from build123d import *

# Parameters (mm, degrees)
F1_DEPTH = 0.6
F3_DEPTH = 1.201


# Not quite as in the source:
# - a feature names something its author has since deleted; it is built from what else it names


with BuildPart() as f1:
    # F0 (on Top) → F1 (new body, symmetric)
    with BuildSketch(Plane.XY):
        Polygon((56, 120), (0, 120), (0, 106), (0, 0), (56, 0), (56, 16), (56, 106), align=None)
        with BuildLine():
            ThreePointArc((62, 100), (57.7573593129, 101.7573593129), (56, 106))
            Line((56, 106), (56, 16))
            ThreePointArc((56, 16), (57.7573593129, 20.2426406871), (62, 22))
            Line((62, 22), (67.5, 22))
            Line((67.5, 22), (67.5, 100))
            Line((67.5, 100), (62, 100))
        make_face()
    extrude(amount=F1_DEPTH, both=True)

    # F2 (on face) → F3 (cut, through all)
    with BuildSketch(Plane.XY.offset(0.6)):
        with BuildLine():
            Line((6, 103), (6, 104.5))
            Line((6, 104.5), (7.5, 104.5))
            ThreePointArc((7.5, 104.5), (4.9393398282, 105.5606601718), (6, 103))
        make_face()
        with BuildLine():
            Line((7.5, 104.5), (6, 104.5))
            Line((6, 104.5), (6, 103))
            ThreePointArc((6, 103), (7.0606601718, 103.4393398282), (7.5, 104.5))
        make_face()
        with BuildLine():
            ThreePointArc((51.5, 104.5), (50, 106), (48.5, 104.5))
            Line((48.5, 104.5), (50, 104.5))
            Line((50, 104.5), (50, 103))
            ThreePointArc((50, 103), (51.0606601718, 103.4393398282), (51.5, 104.5))
        make_face()
        with BuildLine():
            Line((50, 104.5), (48.5, 104.5))
            ThreePointArc((48.5, 104.5), (48.9393398282, 103.4393398282), (50, 103))
            Line((50, 103), (50, 104.5))
        make_face()
        with BuildLine():
            ThreePointArc((51.5, 75.5), (51.0606601718, 76.5606601718), (50, 77))
            Line((50, 77), (50, 75.5))
            Line((50, 75.5), (50, 74))
            ThreePointArc((50, 74), (51.0606601718, 74.4393398282), (51.5, 75.5))
        make_face()
        with BuildLine():
            Line((50, 75.5), (50, 77))
            ThreePointArc((50, 77), (48.5, 75.5), (50, 74))
            Line((50, 74), (50, 75.5))
        make_face()
        with BuildLine():
            ThreePointArc((51.5, 46.5), (51.0606601718, 47.5606601718), (50, 48))
            Line((50, 48), (50, 46.5))
            Line((50, 46.5), (50, 45))
            ThreePointArc((50, 45), (51.0606601718, 45.4393398282), (51.5, 46.5))
        make_face()
        with BuildLine():
            Line((50, 46.5), (50, 48))
            ThreePointArc((50, 48), (48.5, 46.5), (50, 45))
            Line((50, 45), (50, 46.5))
        make_face()
        with BuildLine():
            ThreePointArc((51.5, 17.5), (51.0606601718, 18.5606601718), (50, 19))
            Line((50, 19), (50, 17.5))
            Line((50, 17.5), (48.5, 17.5))
            ThreePointArc((48.5, 17.5), (50, 16), (51.5, 17.5))
        make_face()
        with BuildLine():
            Line((50, 17.5), (50, 19))
            ThreePointArc((50, 19), (48.9393398282, 18.5606601718), (48.5, 17.5))
            Line((48.5, 17.5), (50, 17.5))
        make_face()
        with BuildLine():
            Line((6, 17.5), (6, 19))
            ThreePointArc((6, 19), (4.9393398282, 16.4393398282), (7.5, 17.5))
            Line((7.5, 17.5), (6, 17.5))
        make_face()
        with BuildLine():
            ThreePointArc((7.5, 17.5), (7.0606601718, 18.5606601718), (6, 19))
            Line((6, 19), (6, 17.5))
            Line((6, 17.5), (7.5, 17.5))
        make_face()
        with BuildLine():
            Line((6, 46.5), (6, 48))
            ThreePointArc((6, 48), (4.5, 46.5), (6, 45))
            Line((6, 45), (6, 46.5))
        make_face()
        with BuildLine():
            ThreePointArc((7.5, 46.5), (7.0606601718, 47.5606601718), (6, 48))
            Line((6, 48), (6, 46.5))
            Line((6, 46.5), (6, 45))
            ThreePointArc((6, 45), (7.0606601718, 45.4393398282), (7.5, 46.5))
        make_face()
        with BuildLine():
            Line((6, 75.5), (6, 77))
            ThreePointArc((6, 77), (4.5, 75.5), (6, 74))
            Line((6, 74), (6, 75.5))
        make_face()
        with BuildLine():
            ThreePointArc((7.5, 75.5), (7.0606601718, 76.5606601718), (6, 77))
            Line((6, 77), (6, 75.5))
            Line((6, 75.5), (6, 74))
            ThreePointArc((6, 74), (7.0606601718, 74.4393398282), (7.5, 75.5))
        make_face()
    extrude(amount=-F3_DEPTH, mode=Mode.SUBTRACT)


solid = f1.part
Source: CAD feature listing. Evaluate the final solid. Frame: model axes, mm. Coordinates: 2 decimals unless noted, no trailing zeros. One line per item, written item: value. Start each with the question number.
1. Contact query for a flat-ended pin moving along its axis: P1, Ø0.6, axis at x = 64, z = 0, coming from the +Y side. Output: stop coordinate, or through.
2. Ray query, L1, parallel to Y at x = 6, z = -0.1; L2, parallel to X at y = 17.5, z = 0.3; L3, parallel to X at y = 108, z = -0.35. Return the intervals inside material, ascending.
3. Section A-A (z = 0.15). State how many separate pieces and enclosed holes the cut face has, and give its area (3 significant figures).
Verdict:
1. P1: stops at y = 100
2. L1: y = 0 to 16, 19 to 45, 48 to 74, 77 to 103, 106 to 120
2. L2: x = 0 to 4.5, 7.5 to 48.5, 51.5 to 56.19
2. L3: x = 0 to 56
3. separate pieces: 1
3. enclosed holes: 8
3. area: 7,580 mm2
